Geometry check sheet. Reference: drawing and pictorial views, mm from the part's lowest x, y, z. A direction names the side the tool comes from. Round coordinates to 2 decimals unless told otherwise and drop trailing zeros. Loops run counter-clockwise (first coordinate to the right, second up) from the corner with the lowest first, then second, coordinate; pieces in that order, holes last. Notation, with made-up numbers: M -16,35.25 L 24,35.25 A22 ccw 24,71.25 Z; hole C -31.5,55.25 d3. An arc over 180 degrees is marked long. One line per question, with ' | ' between items. Start each with the question number.
(1) Tool access check on the marked faces 5, 6 and 7. Record the directions out of +Z, -Z, +X, -X, +Y, -Y that give a thin tool (end or side, any length) a straight path to the whole face; none if there is none.
(2) Section check C-C (y = 10.5). Record the boundary of the cut face in (x, z), and give its area (3 significant figures).
(3) Thickness scan on probe 1 along Z at (x, y) = (9.1, 9); probe 2 along Z at (x, y) = (9.1, 10.9); probe 3 along X at (y, z) = (9.75, 31). Record the ranges inside material, lowest first. Write a range as [from, to].
(4) Draft check along Z on the marked faces 1, 2, 3 and 4. Enter one of: +Z half, -Z half, draft (parallel to the pull), parting line (faces both ways), or undercut.
(5) Section check B-B (x = 9.1). Record the boundary of the cut face in (y, z).
(6) Go/stop test with flat-tipped pins: P1, Ø9, axis at x = 9, z = 12, coming from the -Y side; P2, Ø1.5, axis at x = 4, y = 1.5, coming from the +Z side; P3, Ø4, axis at x = 7.5, y = 7, coming from the -Z side; P4, Ø8, axis at x = 3.5, z = 22.5, coming from the -Y side. Record where each tip stops, or that it passes through.
(7) Section check A-A (y = 3). Record the boundary of the cut face in (x, z), and give its area (3 significant figures).
(8) Section check D-D (z = 22.5). Record the boundary of the cut face in (x, y).
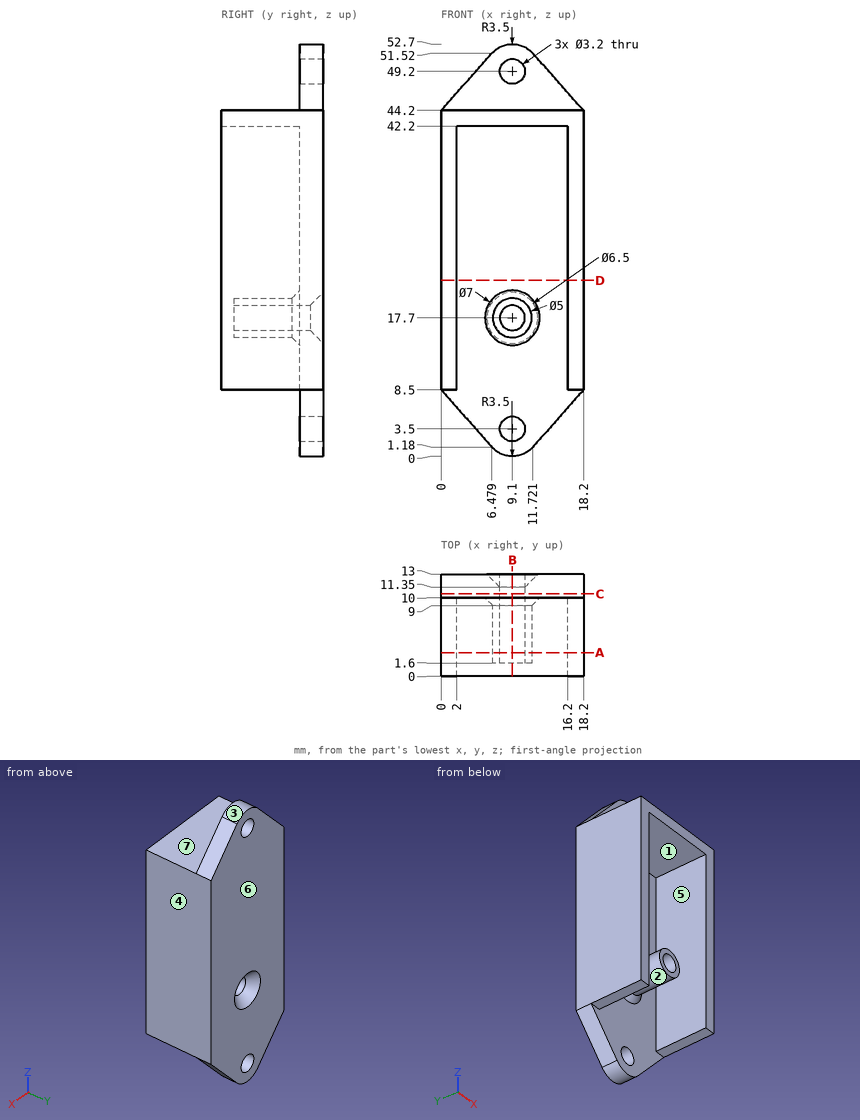
The answers:
1) face 5: -Z, -Y | face 6: +Z, -Z, +X, -X, +Y | face 7: +Z, +X, -X, -Y
2) outline: M 0,8.5 L 6.48,1.18 A3.5 ccw 11.72,1.18 L 18.2,8.5 L 18.2,44.2 L 11.72,51.52 A3.5 ccw 6.48,51.52 L 0,44.2 Z; hole C 9.1,3.5 d3.2; hole C 9.1,17.7 d3.2; hole C 9.1,49.2 d3.2 | area: 806 mm²
3) probe 1: [15.2, 16.1], [19.3, 20.2], [42.2, 44.2] | probe 2: [0, 1.9], [5.1, 16.1], [19.3, 47.6], [50.8, 52.7] | probe 3: [0, 2], [16.2, 18.2]
4) face 1: undercut | face 2: undercut | face 3: +Z half | face 4: draft
5) outline: M 0,42.2 L 10,42.2 L 10,21.2 L 9,20.2 L 1.6,20.2 L 1.6,19.3 L 11.35,19.3 L 13,20.95 L 13,47.6 L 10,47.6 L 10,44.2 L 0,44.2 Z; M 1.6,15.2 L 9,15.2 L 10,14.2 L 10,5.1 L 13,5.1 L 13,14.45 L 11.35,16.1 L 1.6,16.1 Z; M 10,0 L 13,0 L 13,1.9 L 10,1.9 Z; M 10,50.8 L 13,50.8 L 13,52.7 L 10,52.7 Z
6) P1: y = 1.6 | P2: z = 44.2 | P3: z = 15.2 | P4: y = 0
7) outline: M 0,8.5 L 2,8.5 L 2,42.2 L 16.2,42.2 L 16.2,8.5 L 18.2,8.5 L 18.2,44.2 L 0,44.2 Z; C 9.1,17.7 d5; hole C 9.1,17.7 d3.2 | area: 183 mm²
8) outline: M 0,0 L 2,0 L 2,10 L 16.2,10 L 16.2,0 L 18.2,0 L 18.2,13 L 0,13 Z
